Geometry: final body of the model. Coordinates: model frame, mm. Face numbers are marked on the shaded views. A direction names the side the tool comes from. Round coordinates to 2 decimals unless told otherwise and drop trailing zeros. Loops run counter-clockwise (first coordinate to the right, second up) from the corner with the lowest first, then second, coordinate; pieces in that order, holes last. Notation, with made-up numbers: M 37.5,32 L 77.5,32 A26 cw 77.5,58 Z; hole C 51,77.25 d5. An arc over 180 degrees is marked long. Write each question's results on one line, items separated by ' | '.
Autodesk Inventor part; units mm, degrees
ref_plane "YZ Plane" through (0, 0, 0) normal (1, 0, 0) x (0, 1, 0)
ref_plane "XZ Plane" through (0, 0, 0) normal (0, 1, 0) x (-1, 0, 0)
ref_plane "XY Plane" through (0, 0, 0) normal (0, 0, 1) x (1, 0, 0)
sketch "Sketch1" plane through (0, 0, 0) normal (0, 0, 1) x (1, 0, 0)
  line L0 (0, 0) -> (350, 0)
  line L1 (350, 0) -> (350, 200)
  line L2 (350, 200) -> (0, 200)
  line L3 (0, 200) -> (0, 0)
  line L4 (175, 165) -> (175, 35) construction
  line L5 (150, 165) -> (150, 35)
  line L6 (200, 35) -> (200, 165)
  arc A0 (200, 165) -> (150, 165) centre (175, 165) ccw
  arc A1 (150, 35) -> (200, 35) centre (175, 35) ccw
  point P0 (175, 100)
  dimension "d6" = 175
  dimension "d7" = 130
extrude "Extrusion1" add sketch "Sketch1" along normal blind 25
properties part number "disk plate"
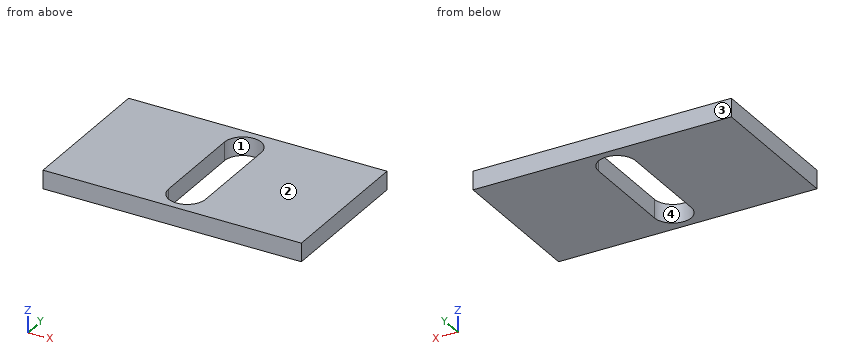
1. Draft query along X for the marked faces 1 and 2. Return one class per face: pulls with the +X half, pulls with the -X half, needs draft (parallel to the pull), parting line crosses it, or undercut.
Answer key:
face 1: undercut | face 2: needs draft
2. Ray query, probe 1 along X at (y, z) = (75, 21.75); probe 2 along X at (y, z) = (13, 13.5); probe 3 along Y at (x, z) = (153, 1.5). Return the intervals inside material, ascending.
Answer key:
probe 1: x = 0 to 150, 200 to 350 | probe 2: x = 0 to 163.13, 186.87 to 350 | probe 3: y = 0 to 23.13, 176.87 to 200
3. Section B-B (y = 94). Output: boundary loops of the cut face in (x, z), then the cut area to 3 significant figures.
Answer key:
outline: M 0,0 L 150,0 L 150,25 L 0,25 Z; M 200,0 L 350,0 L 350,25 L 200,25 Z | area: 7,500 mm²
4. Section C-C (z = 17.75). Output: boundary loops of the cut face in (x, y), then the cut area to 3 significant figures.
Answer key:
outline: M 0,0 L 350,0 L 350,200 L 0,200 Z; hole M 150,35 A25 ccw 200,35 L 200,165 A25 ccw 150,165 Z | area: 61,500 mm²
5. Access query for the marked faces 3 and 4. Directions: +Z, -Z, +X, -X, +Y, -Y. A direction counts if a zero-diameter tool reaches every point of the face in a straight line with its end or side. Return the directions, or none.
Answer key:
face 3: +Z, -Z, +X, -X, +Y | face 4: +Z, -Z
6. Section A-A (x = 175). Output: boundary loops of the cut face in (y, z).
Answer key:
outline: M 0,0 L 10,0 L 10,25 L 0,25 Z; M 190,0 L 200,0 L 200,25 L 190,25 Z
